Could you check a few things on this model? Use its own coordinates, in mm. A direction names the side the tool comes from. Give positions to 0.01 mm unless a question says otherwise; leave off trailing zeros. Write each loop counter-clockwise with the first axis right and the second up, starting at its lowest first coordinate (ties: lowest second). Pieces come first, ordered by that corner, then holes. Notation, with made-up numbers: M 89,72.25 L 99,72.25 A23 cw 99,100.25 Z; hole C 44.5,45 d8. An arc over 180 degrees is marked long. Write each question's results on one line, items separated by ' | '. Start each with the question number.
from build123d import *

# Parameters (mm, degrees)
F1_DEPTH = 3


with BuildPart() as f1:
    # F0 (on Front) → F1 (new body)
    with BuildSketch(Plane.XZ):
        Polygon((-32.600003, -15.6), (-32.600003, -12.6), (-26.300003, -12.6), (-26.300003, -15.6), (-20.000003, -15.6), (-20.000003, -12.6), (-13.700003, -12.6), (-13.700003, -15.6), (-7.400003, -15.6), (-7.400003, -12.6), (-3e-06, -12.6), (-3e-06, -9.6), (-3.000003, -9.6), (-3.000003, -6), (-3e-06, -6), (-3e-06, 0), (-57.900003, 0), (-57.900003, -3), (-60.900003, -3), (-60.900003, 0), (-67.200003, 0), (-67.200003, -3), (-74.600003, -3), (-74.600003, -6), (-71.600003, -6), (-71.600003, -9.6), (-74.600003, -9.6), (-74.600003, -12.6), (-67.200003, -12.6), (-67.200003, -15.6), (-60.900003, -15.6), (-60.900003, -12.6), (-54.600003, -12.6), (-54.600003, -15.6), (-48.300003, -15.6), (-48.300003, -12.6), (-42.000003, -12.6), (-42.000003, -15.6), align=None)
    extrude(amount=F1_DEPTH)


solid = f1.part
Q1. Please list where these lines run through material, in increasing order: line 1 (X direction, y = -2.2, z = -13); line 2 (X direction, y = -1.15, z = -1); line 3 (Z direction, x = -47, y = -1.85). Write a range as [from, to].
Q2. If we section it at B-B (z = -6.75): Please give me the cut outline in (x, y).
Q3. For faces 1 (the face through (-57.9, -1, -1)), 2 (the face through (-4, -1, -12.6)), 3 (the face through (-29, -1, -12.6)), which set-ups out of +Z, -Z, +X, -X, +Y, -Y let a thin tool reach every point of the face, with its end or its side?
Q4. I'm going to push flat-ended pins straight in: P1, Ø1.5, axis at x = -73.5, y = -2, coming from the -Z side; P2, Ø1, axis at x = -56, z = -11, coming from the +Y side; P3, Ø0.9, axis at y = -1, z = -2, coming from the -X side; P4, Ø0.9, axis at x = -71, y = -1, coming from the +Z side. Where does each tip first touch, or does it pass through?
Q5. If we mould it in two halves opening along Z, with no side actions, what happens to faces 4 (the face through (-20, -1, -14)), 5 (the face through (-2, -1, -6)), 6 (the face through (-23, -1, -15.6))? For each: pulls with the +Z half, pulls with the -Z half, needs draft (parallel to the pull), parting line crosses it, or undercut.
Q6. If we section it at A-A (z = -2.25): Please give me the cut outline in (x, y), plus the area to 3 significant figures.
Determined:
1) line 1: x = [-67.2, -60.9], [-54.6, -48.3], [-42, -32.6], [-26.3, -20], [-13.7, -7.4] | line 2: x = [-67.2, -60.9], [-57.9, 0] | line 3: z = [-12.6, 0]
2) outline: M -71.6,-3 L -3,-3 L -3,0 L -71.6,0 Z
3) face 1: +Z, +Y, -Y | face 2: -Z, +X, +Y, -Y | face 3: -Z, +Y, -Y
4) P1: stops at z = -12.6 | P2: stops at y = 0 | P3: stops at x = -67.2 | P4: stops at z = -3
5) face 4: needs draft | face 5: undercut | face 6: pulls with the -Z half
6) outline: M -67.2,-3 L -60.9,-3 L -60.9,0 L -67.2,0 Z; M -57.9,-3 L 0,-3 L 0,0 L -57.9,0 Z | area: 193 mm²
